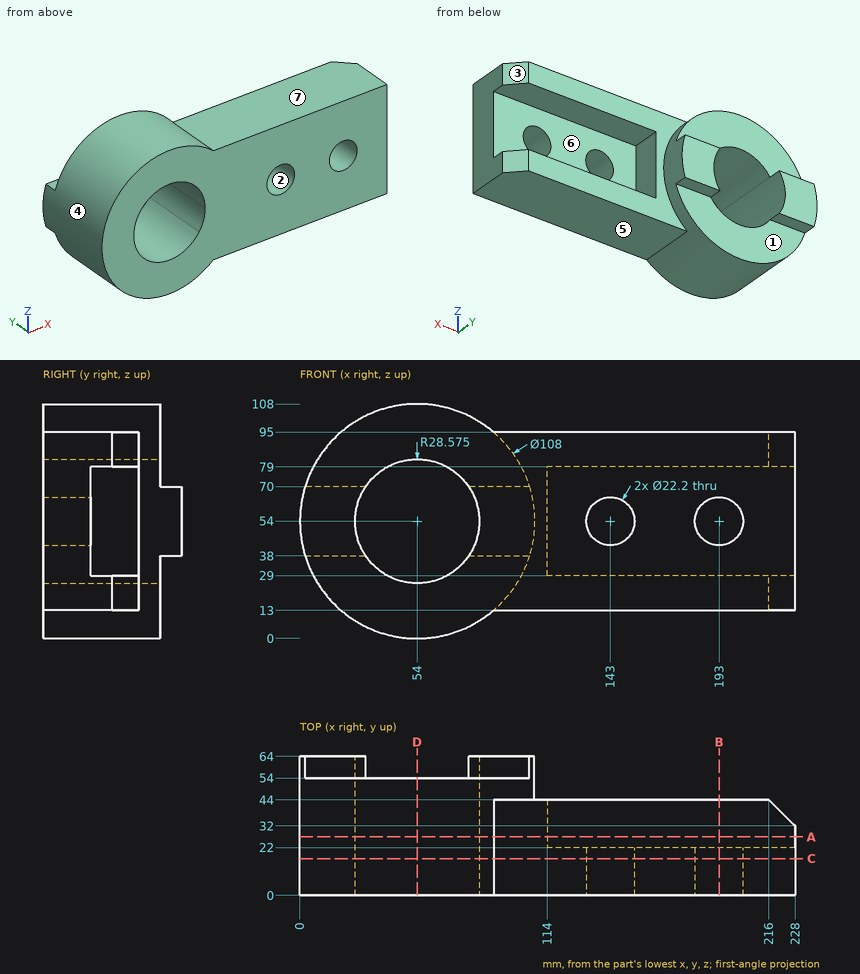
Can you work these out from the drawing? Everything is in mm from the part's minimum corner. A direction names the side the tool comes from. Coordinates: 2 decimals unless noted, no trailing zeros. Loops run counter-clockwise (first coordinate to the right, second up) from the corner with the lowest first, then second, coordinate; pieces in that order, holes last. Notation, with made-up numbers: (35, -33) - (82, -33) arc R16 ccw to (82, -15) - close; hole circle Ø2 at (58.5, 53.25). An arc over 180 degrees is marked (long way). Put each result on its own line as item: value. Start each with the question number.
Item 1: If I drill on line 1 along X through (y, z) = (18, 55); line 2 along Z through (x, y) = (143, 16); line 3 along Y through (x, z) = (52.5, 93), over which ranges is the centre line in solid material (lowest first)?
Item 2: Suppose I cut it at B-B (x = 193). Please give me the cut outline in (y, z), and give its area (3 significant figures).
Item 3: Suppose I cut it at D-D (x = 54). Please give me the cut outline in (y, z) (3 decimals), and give its area (3 significant figures).
Item 4: For pin 1 (17.5 mm diameter, centred on y = 34, z = 46.5, fed in from +X); pin 2 (1 mm diameter, centred on x = 116, y = 41, fed in from +Z); pin 3 (8 mm diameter, centred on y = 12.5, z = 95.5, fed in from -X), each with a flat end and sliding along its axis, tell me the tip position at first contact or that it passes through.
Item 5: Suppose I cut it at A-A (y = 27). Please give me the cut outline in (x, z) (3 decimals), and give its area (3 significant figures).
Item 6: Suppose I cut it at C-C (y = 17). Please give me the cut outline in (x, z) (3 decimals), and give its area (3 significant figures).
Item 7: Which directions (+Z, -Z, +X, -X, +Y, -Y) give clear straight access to the entire face, cutting with the end or side of a thin tool? Please do the marked faces 5, 6 and 7.
Item 8: If we mould it in two halves opening along X, with no side actions, what happens to the marked faces 1, 2, 3 and 4? For each: +X half, -X half, draft (parallel to the pull), parting line (faces both ways), or undercut.
Here are the results:
1. line 1: 0.01 to 25.44, 82.56 to 131.95, 154.05 to 181.95, 204.05 to 228
1. line 2: 13 to 42.9, 65.1 to 95
1. line 3: 0 to 54
2. outline: (0, 13) - (44, 13) - (44, 29) - (22, 29) - (22, 42.9) - (0, 42.9) - close; (0, 65.1) - (22, 65.1) - (22, 79) - (44, 79) - (44, 95) - (0, 95) - close
2. area: 2,020 mm²
3. outline: (0, 0) - (54, 0) - (54, 25.425) - (0, 25.425) - close; (0, 82.575) - (54, 82.575) - (54, 108) - (0, 108) - close
3. area: 2,750 mm²
4. pin 1: x = 114
4. pin 2: z = 95
4. pin 3: x = 15.14
5. outline: (89.143, 13) - (228, 13) - (228, 29) - (114, 29) - (114, 79) - (228, 79) - (228, 95) - (89.143, 95) arc R54 ccw (long way) to start; hole circle Ø57.15 at (54, 54)
5. area: 11,200 mm²
6. outline: (89.143, 13) - (228, 13) - (228, 95) - (89.143, 95) arc R54 ccw (long way) to start; hole circle Ø57.15 at (54, 54); hole circle Ø22.2 at (143, 54); hole circle Ø22.2 at (193, 54)
6. area: 16,100 mm²
7. face 5: -Z, +X, +Y, -Y
7. face 6: +X, +Y
7. face 7: +Z, +X, +Y, -Y
8. face 1: draft
8. face 2: undercut
8. face 3: +X half
8. face 4: parting line
